Can you work these out from the model? Positions are in its coordinate system, mm. Round coordinates to 2 decimals unless told otherwise and drop trailing zeros. Loops run counter-clockwise (first coordinate to the right, second up) from the corner with the lowest first, then second, coordinate; pieces in that order, holes last.
from build123d import *

# Parameters (mm, degrees)
SKETCH2_R                = 3.3
RESSALTO_EXTRUS_O3_DEPTH = 2.5


with BuildPart() as part:
    # Sketch2 → Ressalto-extrusão3 (new, symmetric)
    with BuildSketch(Plane(origin=(0, 0, 0), x_dir=(1, 0, 0), z_dir=(0, 1, 0))):
        with BuildLine():
            Line((41, 93.908069032), (129.747283843, 56.619294308))
            ThreePointArc((129.747283843, 56.619294308), (138.657515974, 49.24995754), (142, 38.180758763))
            Line((142, 38.180758763), (142, 21.025190062))
            ThreePointArc((142, 21.025190062), (140.46792235, 24.627066597), (136.810594171, 26.021601317))
            Line((136.810594171, 26.021601317), (126.810594815, 26.025190062))
            ThreePointArc((126.810594815, 26.025190062), (123.275060909, 24.560723968), (121.810594815, 21.025190062))
            Line((121.810594815, 21.025190062), (121.810594815, -66.724809938))
            ThreePointArc((121.810594815, -66.724809938), (123.275060909, -70.260343844), (126.810594815, -71.724809938))
            Line((126.810594815, -71.724809938), (136.810594815, -71.724809938))
            ThreePointArc((136.810594815, -71.724809938), (140.09446004, -70.495251448), (141.763243519, -67.411301611))
            ThreePointArc((141.763243519, -67.411301611), (135.224391149, -81.092334042), (121.981084486, -88.47759418))
            ThreePointArc((121.981084486, -88.47759418), (120.944283966, -91.984987628), (117.797013197, -93.84817061))
            ThreePointArc((117.797013197, -93.84817061), (117.3987196, -93.882791886), (117, -93.91210234))
            Line((117, -93.91210234), (-117, -93.91210234))
            ThreePointArc((-117, -93.91210234), (-117.3987196, -93.882791886), (-117.797013197, -93.84817061))
            ThreePointArc((-117.797013197, -93.84817061), (-120.944283966, -91.984987628), (-121.981084486, -88.47759418))
            ThreePointArc((-121.981084486, -88.47759418), (-135.224391149, -81.092334042), (-141.763243519, -67.411301611))
            ThreePointArc((-141.763243519, -67.411301611), (-140.09446004, -70.495251448), (-136.810594815, -71.724809938))
            Line((-136.810594815, -71.724809938), (-127, -71.724809938))
            ThreePointArc((-127, -71.724809938), (-123.464466094, -70.260343844), (-122, -66.724809938))
            Line((-122, -66.724809938), (-122, 21.025190062))
            ThreePointArc((-122, 21.025190062), (-123.464466094, 24.560723968), (-127, 26.025190062))
            Line((-127, 26.025190062), (-137, 26.025190062))
            ThreePointArc((-137, 26.025190062), (-140.535533906, 24.560723968), (-142, 21.025190062))
            Line((-142, 21.025190062), (-142, 38.180758763))
            ThreePointArc((-142, 38.180758763), (-138.657515974, 49.24995754), (-129.747283843, 56.619294308))
            Line((-129.747283843, 56.619294308), (-41, 93.908069032))
            Line((-41, 93.908069032), (-41, 81.908069032))
            ThreePointArc((-41, 81.908069032), (-40.121320344, 79.786748689), (-38, 78.908069032))
            Line((-38, 78.908069032), (-25.12, 78.908069032))
            Line((-25.12, 78.908069032), (-25.12, 48.908069032))
            Line((-25.12, 48.908069032), (25.12, 48.908069032))
            Line((25.12, 48.908069032), (25.12, 78.908069032))
            Line((25.12, 78.908069032), (38, 78.908069032))
            ThreePointArc((38, 78.908069032), (40.121320344, 79.786748689), (41, 81.908069032))
            Line((41, 81.908069032), (41, 93.908069032))
        make_face()
        with Locations(Location((-33.06, 15.954790167, 0), (0, 0, 270))):
            Circle(SKETCH2_R, mode=Mode.SUBTRACT)
        with Locations(Location((33.06, 15.954790032, 0), (0, 0, 270))):
            Circle(SKETCH2_R, mode=Mode.SUBTRACT)
        with Locations(Location((33.06, 72.908069032, 0), (0, 0, 270))):
            Circle(SKETCH2_R, mode=Mode.SUBTRACT)
        with Locations(Location((-33.06, 72.908069032, 0), (0, 0, 270))):
            Circle(SKETCH2_R, mode=Mode.SUBTRACT)
        with Locations(Location((-56, 80.908069032, 0), (0, 0, 270))):
            Circle(SKETCH2_R, mode=Mode.SUBTRACT)
        with Locations(Location((-131, 41.025190062, 0), (0, 0, 270))):
            Circle(SKETCH2_R, mode=Mode.SUBTRACT)
        with Locations(Location((56, 80.908069032, 0), (0, 0, 270))):
            Circle(SKETCH2_R, mode=Mode.SUBTRACT)
        with Locations(Location((131, 41.025190062, 0), (0, 0, 270))):
            Circle(SKETCH2_R, mode=Mode.SUBTRACT)
        with Locations(Location((115, -83.974809938, 0), (0, 0, 270))):
            Circle(SKETCH2_R, mode=Mode.SUBTRACT)
        with Locations(Location((-115, -83.908069032, 0), (0, 0, 270))):
            Circle(SKETCH2_R, mode=Mode.SUBTRACT)
    extrude(amount=RESSALTO_EXTRUS_O3_DEPTH, both=True)


solid = part.part
(1) If we section it at D-D, the plane y = 0.7: State how many separate pieces and enclosed holes the cut face has, then the cut area to 3 significant figures.
Worked answers:
separate pieces: 1
enclosed holes: 10
area: 41,600 mm2
(2) If we section it at B-B, the plane z = -15.5: List the corners of the cut face in (x, y) for me, then the cut area to 3 significant figures.
Worked answers:
outline: (-122, -2.5) - (-36.33, -2.5) - (-36.33, 2.5) - (-122, 2.5) - close; (-29.79, -2.5) - (29.79, -2.5) - (29.79, 2.5) - (-29.79, 2.5) - close; (36.33, -2.5) - (121.81, -2.5) - (121.81, 2.5) - (36.33, 2.5) - close
area: 1,150 mm2
(3) If I drill on line 1 (Z direction, x = -13.5, y = 1.75); line 2 (X direction, y = -1.5, z = 16); line 3 (X direction, y = -1.4, z = -56.5), over which ranges is the centre line in solid material (lowest first)?
Worked answers:
line 1: z = -48.91 to 93.91
line 2: x = -122 to 121.81
line 3: x = -130.03 to -25.12, 25.12 to 130.03
(4) If we section it at C-C, the plane x = 56: List the corners of the cut face in (y, z) for me, then the cut area to 3 significant figures.
Worked answers:
outline: (-2.5, -87.61) - (2.5, -87.61) - (2.5, -84.21) - (-2.5, -84.21) - close; (-2.5, -77.61) - (2.5, -77.61) - (2.5, 93.91) - (-2.5, 93.91) - close
area: 875 mm2
(5) If we section it at A-A, the plane x = -33.06: List the corners of the cut face in (y, z) for me.
Worked answers:
outline: (-2.5, -78.91) - (2.5, -78.91) - (2.5, -76.21) - (-2.5, -76.21) - close; (-2.5, -69.61) - (2.5, -69.61) - (2.5, -19.25) - (-2.5, -19.25) - close; (-2.5, -12.65) - (2.5, -12.65) - (2.5, 93.91) - (-2.5, 93.91) - close
(6) If we mould it in two halves opening along X, with no side actions, what happens to faces 1 (the cylindrical face through (127.78, -0.04, -41.74)), 2 (the cylindrical face through (-35.07, -0.04, -18.57)), 3 (the flat face through (2, 2.5, 20)), 4 (the flat face through (-86, 0, -75))? For each: released by +X, released by -X, zero draft, split by the parting line, or undercut.
Worked answers:
face 1: undercut
face 2: undercut
face 3: zero draft
face 4: released by -X
(7) Will this pin go through, and if not, where does the flat tip stop? P1, Ø2.5, axis at y = -0.5, z = 22, coming from the -X side.
Worked answers:
P1: stops at x = -122
